```python
from build123d import *

# Parameters (mm, degrees)
F1_DEPTH     = 25.4
F2_R         = 3.556
F3_DEPTH     = 17.78
F4_R         = 9.525
F4_R_2       = 3.556
F5_DEPTH     = 7.62
F6_T1_DEPTH  = 48.26
F6_T3_DEPTH  = 20.828
F6_T5_DEPTH  = 15.24
F6_S9_W      = 5.08
F6_S9_H      = 5.08
F6_T10_DEPTH = 5.08
F6_S15_W     = 5.08
F6_S15_H     = 5.08
F6_T16_DEPTH = 5.08
F7_SIZE      = 5.07999
F8_R         = 5.08
F9_T3_DEPTH  = 15.24
F9_T6_DEPTH  = 11.413497326
F9_T10_DEPTH = 11.413497326
F9_T14_ANGLE = 89.9999999979
F9_T17_ANGLE = 89.9999999979


# Not quite as in the source:
# - a fillet or chamfer that OpenCascade refuses, or shapes differently, is made with other operations: its cross-section is extruded or revolved along the edge and cut away or added
# - a fillet or chamfer is up to 0.001 mm smaller than in the source, because OpenCascade refuses the exact size


with BuildPart() as f1:
    # F0 (on Right) → F1 (new body)
    with BuildSketch(Plane.YZ):
        with BuildLine():
            Line((0, -25.4), (0, 0))
            Line((0, 0), (-4.572, 0))
            ThreePointArc((-4.572, 0), (-6.858, 2.286), (-4.572, 4.572))
            Line((-4.572, 4.572), (-4.572, 15.24))
            Line((-4.572, 15.24), (-17.78, 15.24))
            Line((-17.78, 15.24), (-17.78, 0))
            Line((-17.78, 0), (-17.78, -25.4))
            Line((-17.78, -25.4), (0, -25.4))
        make_face()
    extrude(amount=F1_DEPTH)

    # F2 (on face) → F3 (cut, through all)
    with BuildSketch(Plane(origin=(0, 0, 0), x_dir=(-1, 0, 0), z_dir=(0, 1, 0))):
        with Locations((-12.7, -5.08)):
            Circle(F2_R)
    extrude(amount=-F3_DEPTH, mode=Mode.SUBTRACT)

    # F4 (on face) → F5 (cut)
    with BuildSketch(Plane.XZ.offset(17.78)):
        with Locations((12.7, -5.08)):
            Circle(F4_R)
        with Locations((12.7, -5.08)):
            Circle(F4_R_2, mode=Mode.SUBTRACT)
    extrude(amount=-F5_DEPTH, mode=Mode.SUBTRACT)

    # F6: fillet of radius 5.08 on 5 edges, made by hand

    # F6_s2 → F6_t1 (cut)
    with BuildSketch(Plane.XY.offset(-38.1)):
        with BuildLine():
            ThreePointArc((5.08, -17.78), (1.4878975516, -16.2921024484), (0, -12.7))
            Line((0, -12.7), (0, -17.78))
            Line((0, -17.78), (5.08, -17.78))
        make_face()
        with BuildLine():
            ThreePointArc((20.32, -17.78), (23.9121024484, -16.2921024484), (25.4, -12.7))
            Line((25.4, -12.7), (25.4, -17.78))
            Line((25.4, -17.78), (20.32, -17.78))
        make_face()
    extrude(amount=F6_T1_DEPTH, mode=Mode.SUBTRACT)

    # F6_s4 → F6_t3 (cut)
    with BuildSketch(Plane.XZ.offset(-8.128)):
        with BuildLine():
            ThreePointArc((20.32, 15.24), (23.9121024484, 13.7521024484), (25.4, 10.16))
            Line((25.4, 10.16), (25.4, 15.24))
            Line((25.4, 15.24), (20.32, 15.24))
        make_face()
        with BuildLine():
            ThreePointArc((5.08, 15.24), (1.4878975516, 13.7521024484), (0, 10.16))
            Line((0, 10.16), (0, 15.24))
            Line((0, 15.24), (5.08, 15.24))
        make_face()
    extrude(amount=F6_T3_DEPTH, mode=Mode.SUBTRACT)

    # F6_s6 → F6_t5 (cut)
    with BuildSketch(Plane.YZ.offset(5.08)):
        with BuildLine():
            ThreePointArc((-17.78, 10.16), (-16.2921024484, 13.7521024484), (-12.7, 15.24))
            Line((-12.7, 15.24), (-17.78, 15.24))
            Line((-17.78, 15.24), (-17.78, 10.16))
        make_face()
    extrude(amount=F6_T5_DEPTH, mode=Mode.SUBTRACT)


with BuildPart() as f6_tool8:
    # F6_s9 → F6_t10 (new body)
    with BuildSketch(Plane.YZ.offset(5.08)):
        with Locations((-15.24, 12.7)):
            Rectangle(F6_S9_W, F6_S9_H)
    extrude(amount=-F6_T10_DEPTH)

    # F6_s11 → F6_t12 (revolve, cut)
    with BuildSketch(Plane(origin=(5.08, -12.7, 10.16), x_dir=(0, 0.7071067812, -0.7071067812), z_dir=(0, 0.7071067812, 0.7071067812))):
        with BuildLine():
            ThreePointArc((0, -5.08), (5.08, 0), (0, 5.08))
            Line((0, 5.08), (0, -5.08))
        make_face()
    revolve(axis=Axis((5.08, -12.7, 10.16), (-1, 0, 0)), mode=Mode.SUBTRACT)


with BuildPart() as f1_1:
    add(f1.part)

    # F6_t7: cut F6_tool8
    add(f6_tool8.part, mode=Mode.SUBTRACT)


with BuildPart() as f6_tool14:
    # F6_s15 → F6_t16 (new body)
    with BuildSketch(Plane.YZ.offset(20.32)):
        with Locations((-15.24, 12.7)):
            Rectangle(F6_S15_W, F6_S15_H)
    extrude(amount=F6_T16_DEPTH)

    # F6_s17 → F6_t18 (revolve, cut)
    with BuildSketch(Plane(origin=(20.32, -12.7, 10.16), x_dir=(0, 0.7071067812, -0.7071067812), z_dir=(0, -0.7071067812, -0.7071067812))):
        with BuildLine():
            ThreePointArc((0, -5.08), (5.08, 0), (0, 5.08))
            Line((0, 5.08), (0, -5.08))
        make_face()
    revolve(axis=Axis((20.32, -12.7, 10.16), (1, 0, 0)), mode=Mode.SUBTRACT)


with BuildPart() as f1_2:
    add(f1_1.part)

    # F6_t13: cut F6_tool14
    add(f6_tool14.part, mode=Mode.SUBTRACT)

    # F7 (size 5.08 in the source; OpenCascade refuses exactly that, so slightly less here)
    f7_edges = [f1_2.edges().sort_by_distance(p)[0] for p in [
        (12.7, -17.78, -25.4),
    ]]
    chamfer(f7_edges, length=F7_SIZE)

    # F8
    f8_edges = [f1_2.edges().sort_by_distance(p)[0] for p in [
        (12.7, -17.78, -20.32001),
        (0, -6.35, -20.32001),
        (25.4, -6.35, -20.32001),
        (1.487898, -16.292102, -20.32001),
        (23.912102, -16.292102, -20.32001),
    ]]
    fillet(f8_edges, radius=F8_R)

    # F9: fillet of radius 2.3301989304 on 5 edges, made by hand


with BuildPart() as f9_tool1:
    # F9_s2 → F9_t3 (new body)
    with BuildSketch(Plane.YZ.offset(5.08)):
        with BuildLine():
            ThreePointArc((-4.572, 12.9098010696), (-5.2544994652, 14.5575005348), (-6.9021989304, 15.24))
            Line((-6.9021989304, 15.24), (-4.572, 15.24))
            Line((-4.572, 15.24), (-4.572, 12.9098010696))
        make_face()
    extrude(amount=F9_T3_DEPTH)


with BuildPart() as f9_tool4:
    # F9_s5 → F9_t6 (new body)
    with BuildSketch(Plane.XY.offset(-1.253497326)):
        with BuildLine():
            ThreePointArc((0, -6.9021989304), (0.6824994652, -5.2544994652), (2.3301989304, -4.572))
            Line((2.3301989304, -4.572), (0, -4.572))
            Line((0, -4.572), (0, -6.9021989304))
        make_face()
    extrude(amount=F9_T6_DEPTH)

    split(bisect_by=Plane.XY, keep=Keep.TOP)


with BuildPart() as f9_tool8:
    # F9_s9 → F9_t10 (new body)
    with BuildSketch(Plane.XY.offset(-1.253497326)):
        with BuildLine():
            ThreePointArc((25.4, -6.9021989304), (24.7175005348, -5.2544994652), (23.0698010696, -4.572))
            Line((23.0698010696, -4.572), (25.4, -4.572))
            Line((25.4, -4.572), (25.4, -6.9021989304))
        make_face()
    extrude(amount=F9_T10_DEPTH)

    split(bisect_by=Plane.XY, keep=Keep.TOP)


with BuildPart() as f9_tool12:
    # F9_s13 → F9_t14 (revolve)
    with BuildSketch(Plane.XY.offset(10.1599999999)):
        with BuildLine():
            ThreePointArc((0, -6.9021989304), (0.6824994652, -5.2544994652), (2.3301989304, -4.572))
            Line((2.3301989304, -4.572), (0, -4.572))
            Line((0, -4.572), (0, -6.9021989304))
        make_face()
    revolve(axis=Axis((5.0800000001, -4.572, 10.1599999999), (0, 1, 0)), revolution_arc=F9_T14_ANGLE)


with BuildPart() as f9_tool15:
    # F9_s16 → F9_t17 (revolve)
    with BuildSketch(Plane.YZ.offset(20.3199999999)):
        with BuildLine():
            ThreePointArc((-4.572, 12.9098010696), (-5.2544994652, 14.5575005348), (-6.9021989304, 15.24))
            Line((-6.9021989304, 15.24), (-4.572, 15.24))
            Line((-4.572, 15.24), (-4.572, 12.9098010696))
        make_face()
    revolve(axis=Axis((20.3199999999, -4.572, 10.1599999999), (0, 1, 0)), revolution_arc=F9_T17_ANGLE)


with BuildPart() as f1_3:
    add(f1_2.part)

    # F9_t18: cut F9_tool1, F9_tool4, F9_tool8, F9_tool12, F9_tool15
    add([f9_tool1.part, f9_tool4.part, f9_tool8.part, f9_tool12.part, f9_tool15.part], mode=Mode.SUBTRACT)


solid = f1_3.part
```
Can you work these out from the model? Positions are in its coordinate system, mm. A direction names the side the tool comes from. Coordinates: 2 decimals unless noted, no trailing zeros. Loops run counter-clockwise (first coordinate to the right, second up) from the corner with the lowest first, then second, coordinate; pieces in that order, holes last. Notation, with made-up numbers: (37.5, 88) -> (82.5, 88) arc R9 cw to (82.5, 95) -> close; hole circle Ø4 at (22, 31.5). An arc over 180 degrees is marked (long way). Answer as a JSON object with one key per item and string values.
1) If I drill on line 1 (Z direction, x = 12.7, y = -2.75); line 2 (X direction, y = -3, z = -5.08); line 3 (Z direction, x = 12.7, y = -12) (3 decimals), over which ranges is the centre line in solid material (lowest first)?
Results:
{"line 1": "z = -25.4 to -8.64, -1.52 to 0", "line 2": "x = 0 to 9.14, 16.26 to 25.4", "line 3": "z = -25.4 to -14.605, 4.445 to 15.24"}
2) For faces 5 (the face through (13, -4.572, 9)), 6 (the face through (1.528, -16.331, -4.227)), 7 (the face through (24.736, -5.273, 7.267)), which set-ups out of +Z, -Z, +X, -X, +Y, -Y let a thin tool reach every point of the face, with its end or its side?
Results:
{"face 5": "+Z, +X, -X, +Y", "face 6": "+Z, -Z, -X, -Y", "face 7": "+Z, +X, +Y"}
3) Imagine slicing it at B-B (z = 7). Please give me the cut outline in (x, y), then the cut area to 3 significant figures.
Results:
{"outline": "(0, -12.7) arc R5.08 ccw to (5.08, -17.78) -> (20.32, -17.78) arc R5.08 ccw to (25.4, -12.7) -> (25.4, -6.9) arc R2.33 ccw to (23.07, -4.57) -> (2.33, -4.57) arc R2.33 ccw to (0, -6.9) -> close", "area": "322 mm^2"}
4) Imagine slicing it at C-C (y = -9.75). Please give me the cut outline in (x, z).
Results:
{"outline": "(0, -18.22) arc R5.08 ccw to (1.49, -21.81) -> (5.08, -25.4) -> (20.32, -25.4) -> (23.91, -21.81) arc R5.08 ccw to (25.4, -18.22) -> (25.4, 10.16) arc R5.08 ccw to (20.32, 15.24) -> (5.08, 15.24) arc R5.08 ccw to (0, 10.16) -> close; hole circle Ø7.11 at (12.7, -5.08)"}
5) Imagine slicing it at D-D (z = -5.08). Please give me the cut outline in (x, y) (3 decimals), then the cut area to 3 significant figures.
Results:
{"outline": "(0, -12.7) arc R5.08 ccw to (3.175, -17.409) -> (3.175, -10.16) -> (9.144, -10.16) -> (9.144, 0) -> (0, 0) -> close; (16.256, -10.16) -> (22.225, -10.16) -> (22.225, -17.409) arc R5.08 ccw to (25.4, -12.7) -> (25.4, 0) -> (16.256, 0) -> close", "area": "224 mm^2"}
6) Thinking about a two-plate mould opening in Z: for faces 1 (the face through (12.522, -6.857, 2.236)), 2 (the face through (13, -10, 15.24)), 3 (the face through (17, -10.16, -5)), 4 (the face through (0.4, -6.44, -20.19)), which applies, pulls with the +Z half, pulls with the -Z half, needs draft (parallel to the pull), parting line crosses it, or undercut?
Results:
{"face 1": "undercut", "face 2": "pulls with the +Z half", "face 3": "undercut", "face 4": "pulls with the -Z half"}
7) Imagine slicing it at A-A (x = 12.7). Please give me the cut outline in (y, z) (3 decimals), then the cut area to 3 significant figures.
Results:
{"outline": "(-17.78, -18.216) arc R5.08 ccw to (-16.292, -21.808) -> (-12.7, -25.4) -> (0, -25.4) -> (0, -8.636) -> (-10.16, -8.636) -> (-10.16, -14.605) -> (-17.78, -14.605) -> close; (-17.78, 4.445) -> (-10.16, 4.445) -> (-10.16, -1.524) -> (0, -1.524) -> (0, 0) -> (-4.572, 0) arc R2.286 cw to (-4.572, 4.572) -> (-4.572, 12.91) arc R2.33 ccw to (-6.902, 15.24) -> (-12.7, 15.24) arc R5.08 ccw to (-17.78, 10.16) -> close", "area": "407 mm^2"}
8) For P1, Ø5.5, axis at x = 16, z = -7, coming from the -Y side; P2, Ø11.5, axis at x = 12.7, z = -5.08, coming from the +Y side; P3, Ø9, axis at x = 14, z = 9, coming from the +Y side; P4, Ø5.5, axis at x = 14.5, y = -2.5, coming from the +Z side, each with a flat end and sliding along its axis, tell me the tip position at first contact or that it passes through.
Results:
{"P1": "stops at y = -10.16", "P2": "stops at y = 0", "P3": "stops at y = -4.57", "P4": "stops at z = 14.55"}
